from build123d import *

# Parameters (mm, degrees)
BOSS_EXTRUDE1_DEPTH = 29
SKETCH2_R           = 2
SKETCH2_R_2         = 1.5
CUT_EXTRUDE1_DEPTH  = 10
SKETCH3_R           = 2.75
CUT_EXTRUDE2_DEPTH  = 6
DRAFT1_ANGLE        = 5


with BuildPart() as part:
    # Sketch1 → Boss-Extrude1 (new body)
    with BuildSketch(Plane(origin=(0, 0, 0), x_dir=(1, 0, 0), z_dir=(0, 1, 0))):
        Polygon((10.420353982, -7.201327434), (-4.579646018, -7.201327434), (-4.579646018, 7.798672566), (-0.312469404, 7.798672566), (10.420353982, -0.201327434), align=None)
    extrude(amount=BOSS_EXTRUDE1_DEPTH)

    # Sketch2 → Cut-Extrude1 (cut)
    with BuildSketch(Plane.XZ):
        with Locations(Location((-0.579646018, 2.201327434, 0), (0, 0, 270))):
            Circle(SKETCH2_R)
        with Locations(Location((7.420353982, 2.201327434, 0), (0, 0, 270))):
            Circle(SKETCH2_R_2)
    extrude(amount=-CUT_EXTRUDE1_DEPTH, mode=Mode.SUBTRACT)

    # Sketch3 → Cut-Extrude2 (cut)
    with BuildSketch(Plane(origin=(0, 29, 0), x_dir=(1, 0, 0), z_dir=(0, 1, 0))):
        with Locations(Location((3.420353982, -0.201327434, 0), (0, 0, 270))):
            Circle(SKETCH3_R)
    extrude(amount=-CUT_EXTRUDE2_DEPTH, mode=Mode.SUBTRACT)

    # Draft1
    draft1_faces = [part.faces().sort_by_distance(p)[0] for p in [
        (5.053942289, 14.5, -3.798672566),
        (-2.446057711, 14.5, -7.798672566),
        (-4.579646018, 14.5, -0.298672566),
        (10.420353982, 14.5, 3.701327434),
        (2.920353982, 14.5, 7.201327434),
    ]]
    draft(draft1_faces, Plane.ZX.offset(29), DRAFT1_ANGLE)


solid = part.part
For this review, take the finished solid that the model builds, in its own axes (mm). A direction names the side the tool comes from. Round coordinates to 2 decimals unless told otherwise and drop trailing zeros. Loops run counter-clockwise (first coordinate to the right, second up) from the corner with the lowest first, then second, coordinate; pieces in that order, holes last. Notation, with made-up numbers: (4.25, -12.75) - (53.25, -12.75) arc R12 cw to (53.25, -2.75) - close; hole circle Ø9 at (-24, 69). An arc over 180 degrees is marked (long way). Put each result on its own line as item: value. Start each with the question number.
1. Consider section C-C on z = 5.25. State the section outline as (x, y) points.
2. Consider section D-D on y = 23.5. State the section outline as (x, z) points.
3. Mouldability with a two-part tool opening along Z and no side actions: class faces 4 (the flat face through (3, 23, 0)), 5 (the flat face through (1, 29, 3)), 6 (the flat face through (-2.498, 11.075, -9.367)), 7 (the flat face through (3.061, 14.297, 8.488)) as +Z half, -Z half, draft (parallel to the pull), parting line (faces both ways), or undercut.
4. Consider section A-A on y = 9. State the section outline as (x, z) points.
5. For faces 1 (the cylindrical face through (-0.5, 4.9, 4.2)), 2 (the flat face through (3, 0, 0)), 3 (the cylindrical face through (5.74, 26.04, 1.68)), list the 3-axis set-ups (+Z, -Z, +X, -X, +Y, -Y) from which the entire face can be reached by the end or side of a thin tool; tool diameter is ignored.
6. For probe 1 along X at (y, z) = (23.5, 1.25); probe 2 along Y at (x, z) = (2.5, -1); probe 3 along Z at (x, y) = (-1, 8.25), list the stretches that pass through material, from the lowest coordinate up. Write a range as [from, to].
7. Consider section B-B on x = 4.25. State the section outline as (y, z) points, plus the area to 3 significant figures.
8. Insertion check: P1, Ø3.5, axis at x = -0.58, z = 2.2, coming from the -Y side; P2, Ø2, axis at x = 3, y = 24.5, coming from the -Z side; P3, Ø4, axis at x = 11, y = 11.5, coming from the +Z side. Each pin has a flat end and moves straight along its axis. Give the tip position at first contact, or say it passes through.
Result sheet:
1. outline: (-7.12, 0) - (12.96, 0) - (10.42, 29) - (-4.58, 29) - close
2. outline: (-5.06, -8.28) - (-0.15, -8.28) - (10.9, -0.04) - (10.9, 7.68) - (-5.06, 7.68) - close; hole circle Ø5.5 at (3.42, 0.2)
3. face 4: undercut
3. face 5: draft
3. face 6: -Z half
3. face 7: +Z half
4. outline: (-6.33, -9.55) - (0.27, -9.55) - (12.17, -0.68) - (12.17, 8.95) - (-6.33, 8.95) - close; hole circle Ø4 at (-0.58, 2.2); hole circle Ø3 at (7.42, 2.2)
5. face 1: -Y
5. face 2: +Z, -Z, +X, -X, -Y
5. face 3: +Y
6. probe 1: [-5.06, 0.88], [5.96, 10.9]
6. probe 2: [0, 23]
6. probe 3: [-9.61, 0.25], [4.16, 9.02]
7. outline: (0, -7.56) - (29, -4.4) - (29, -2.42) - (23, -2.42) - (23, 2.82) - (29, 2.82) - (29, 7.2) - (0, 9.74) - close
7. area: 388 mm^2
8. P1: y = 10
8. P2: z = -6.57
8. P3: z = 8.91
